Study the drawing (mm; zero at the part's minimum x, y, z) and answer. A direction names the side the tool comes from. Give positions to 0.01 mm unless a question says otherwise; leave off trailing zeros. Write each loop counter-clockwise with the first axis right and the second up, starting at its lowest first coordinate (ties: lowest second). Pieces come first, ordered by that corner, then holes. Notation, with made-up numbers: (64, -34) - (108, -34) arc R13 ccw to (108, -20) - close; hole circle Ø2 at (6, 41.25). An arc over 180 degrees is marked (long way). Return JSON: item names as keys, results as strings.
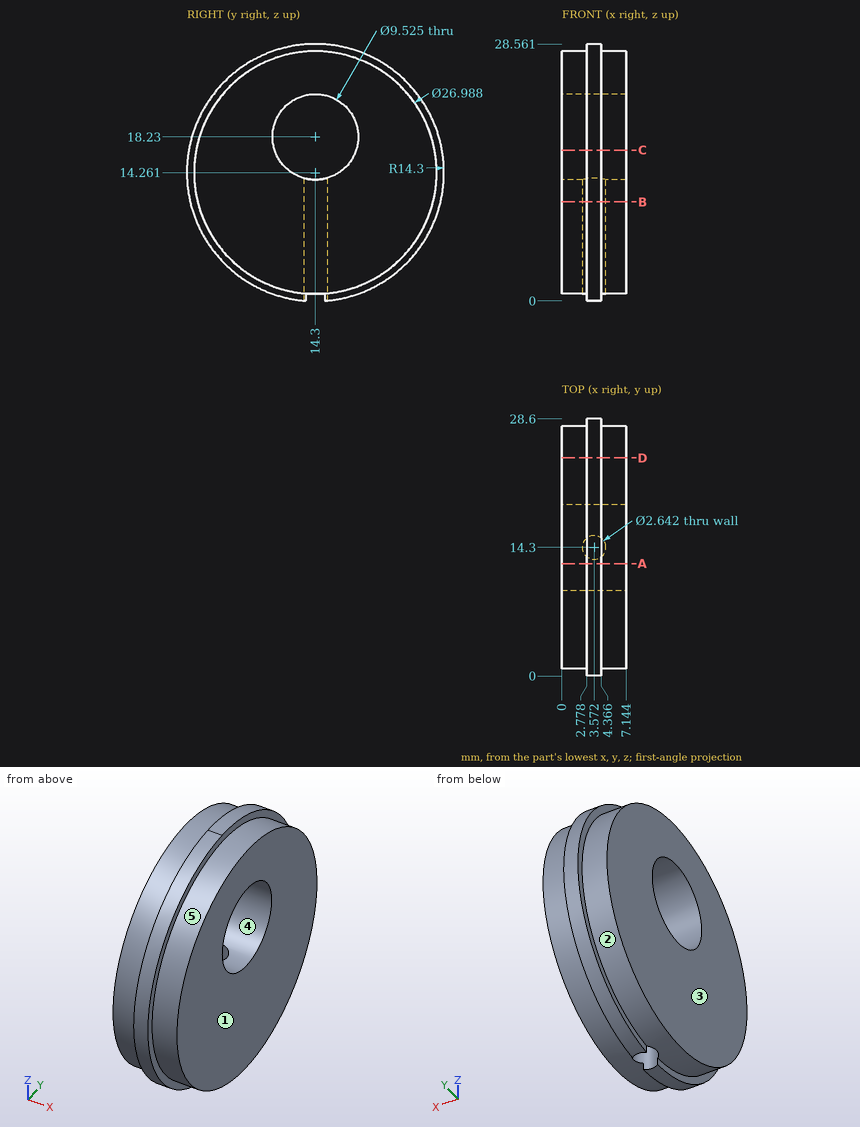
Item 1: A cutting plane is placed at C-C on z = 16.75. Determine the outline of the cut face in (x, y) (1 decimal).
Answer below:
{"outline": "(0, 1) - (2.8, 1) - (2.8, 0.2) - (4.4, 0.2) - (4.4, 1) - (7.1, 1) - (7.1, 9.8) - (0, 9.8) - close; (0, 18.8) - (7.1, 18.8) - (7.1, 27.6) - (4.4, 27.6) - (4.4, 28.4) - (2.8, 28.4) - (2.8, 27.6) - (0, 27.6) - close"}
Item 2: Consider L1, parallel to Z at x = 5.25, y = 12 (1 decimal); L2, parallel to Z at x = 6, y = 13.5 (1 decimal); L3, parallel to Y at x = 5.25, z = 19.5 (1 decimal). Determine where each line is inside the solid, lowest interval first.
Answer below:
{"L1": "z = 1 to 14.1, 22.4 to 27.6", "L2": "z = 0.8 to 13.5, 22.9 to 27.7", "L3": "y = 1.9 to 9.7, 18.9 to 26.7"}
Item 3: A cutting plane is placed at B-B on z = 11. Determine the outline of the cut face in (x, y) (1 decimal), then the cut area to 3 significant figures.
Answer below:
{"outline": "(0, 1.2) - (2.8, 1.2) - (2.8, 0.4) - (4.4, 0.4) - (4.4, 1.2) - (7.1, 1.2) - (7.1, 27.4) - (4.4, 27.4) - (4.4, 28.2) - (2.8, 28.2) - (2.8, 27.4) - (0, 27.4) - close; hole circle Ø2.6 at (3.6, 14.3)", "area": "184 mm²"}
Item 4: For the marked faces 1 and 2, determine the directions among +Z, -Z, +X, -X, +Y, -Y from which every point of the face is accessible in a straight line to the end or side of a thin tool.
Answer below:
{"face 1": "+Z, -Z, +X, +Y, -Y", "face 2": "-X"}
Item 5: Flat-ended cylindrical pins translate along their axes: P1, Ø1, axis at x = 6, y = 10, coming from the +Z side; P2, Ø1, axis at x = 5.5, z = 22, coming from the +Y side; P3, Ø4, axis at x = 3, z = 24, coming from the -Y side (1 decimal). Find the tip coordinate at first contact, or state that the pin passes through.
Answer below:
{"P1": "stops at z = 27.21", "P2": "stops at y = 25.69", "P3": "stops at y = 2.3"}
Item 6: The mould has two halves that part along Y. Classify the marked faces 3, 4 and 5: +Y half, -Y half, draft (parallel to the pull), parting line (faces both ways), or undercut.
Answer below:
{"face 3": "draft", "face 4": "undercut", "face 5": "parting line"}
Item 7: A cutting plane is placed at D-D on y = 24.25. Determine the outline of the cut face in (x, z) (1 decimal).
Answer below:
{"outline": "(0, 5.1) - (2.8, 5.1) - (2.8, 4) - (4.4, 4) - (4.4, 5.1) - (7.1, 5.1) - (7.1, 23.4) - (4.4, 23.4) - (4.4, 24.5) - (2.8, 24.5) - (2.8, 23.4) - (0, 23.4) - close"}
Item 8: A cutting plane is placed at A-A on y = 12.5. Determine the outline of the cut face in (x, z) (1 decimal).
Answer below:
{"outline": "(0, 0.9) - (2.8, 0.9) - (2.8, 0.1) - (4.4, 0.1) - (4.4, 0.9) - (7.1, 0.9) - (7.1, 13.8) - (0, 13.8) - close; (0, 22.6) - (7.1, 22.6) - (7.1, 27.6) - (4.4, 27.6) - (4.4, 28.4) - (2.8, 28.4) - (2.8, 27.6) - (0, 27.6) - close"}
